Here's how the part is built. I have some questions about the finished solid (model axes, mm). A direction names the side the tool comes from. Coordinates: 2 decimals unless noted, no trailing zeros. Write each loop counter-clockwise with the first axis right and the second up, starting at its lowest first coordinate (ties: lowest second). Pieces come first, ordered by that corner, then holes.
Item 1: If we section it at A-A (x = -8): Please give me the cut outline in (y, z).
Item 2: For faces 5 (the face through (-11, 13, 3.6)), 6 (the face through (9.33, 31.864, 5.215)), 7 (the face through (15, 15, 4)), 8 (the face through (14, -6.48, 0.4)), 9 (the face through (5.75, 13, 2)), which set-ups out of +Z, -Z, +X, -X, +Y, -Y let a thin tool reach every point of the face, with its end or its side?
Item 3: I'm going to push flat-ended pins straight in: pin 1 Ø2 at (y, z) = (33.5, 5) entering from +X; pin 2 Ø1.5 at (x, y) = (9, 25) entering from -Z; pin 3 Ø3 at (y, z) = (33.5, 5) entering from +X. Where does each tip first touch, or does it pass through?
Item 4: If we section it at B-B (y = 7): Please give me the cut outline in (x, z).
Item 5: If I drill on line 1 (X direction, y = 16, z = 1); line 2 (Y direction, x = 8, z = 5); line 3 (X direction, y = 14.5, z = 7), over which ranges is the centre line in solid material (lowest first)?
Item 6: We'd pull the mould along Y, two halves only. Please class faces 1 (the face through (-14.43, -6.9, 3.96)), 2 (the face through (-4, 13, 6)), 3 (the face through (4, 13, 6)), 4 (the face through (-14.5, 14.7, 0.5)): +Y half, -Y half, draft (parallel to the pull), parting line (faces both ways), or undercut.
Item 7: If we section it at C-C (x = 9): Please give me the cut outline in (y, z).
from build123d import *

# Parameters (mm, degrees)
SKETCH1_W           = 30
SKETCH1_H           = 75
BOSS_EXTRUDE1_DEPTH = 8
FILLET2_R           = 2
CUT_EXTRUDE3_DEPTH  = 4.4
CUT_EXTRUDE4_DEPTH  = 4.4
SKETCH11_W          = 30
SKETCH11_H          = 30
CUT_EXTRUDE5_DEPTH  = 29.4
FILLET3_R           = 2
CHAMFER1_SIZE       = 1


with BuildPart() as part:
    # Sketch1 → Boss-Extrude1 (new body)
    with BuildSketch(Plane.XY):
        Rectangle(SKETCH1_W, SKETCH1_H)
    extrude(amount=BOSS_EXTRUDE1_DEPTH)

    # Sketch3 → M4 Tapped Hole1 (revolve, cut)
    with BuildSketch(Plane(origin=(15, 33.5, 5), x_dir=(0, 0, -1), z_dir=(0, 1, 0))):
        Polygon((0, 0), (0, 12.491420021), (1.65, 11.5), (1.65, 0), align=None)
    m4_tapped_hole1 = revolve(axis=Axis((21.35, 33.5, 5), (-1, 0, 0)), mode=Mode.SUBTRACT)

    # Fillet2
    fillet2_edges = [part.edges().sort_by_distance(p)[0] for p in [
        (0, 37.5, 0),
        (0, 37.5, 8),
    ]]
    fillet(fillet2_edges, radius=FILLET2_R)

    # Sketch9 → Cut-Extrude3 (cut)
    with BuildSketch(Plane.XY.offset(8)):
        with BuildLine():
            Line((-12, 0), (-12, 25))
            ThreePointArc((-12, 25), (-8, 29), (-4, 25))
            Line((-4, 25), (-4, 0))
            ThreePointArc((-4, 0), (-8, -4), (-12, 0))
        make_face()
        with BuildLine():
            Line((12, 0), (12, 25))
            ThreePointArc((12, 25), (8, 29), (4, 25))
            Line((4, 25), (4, 0))
            ThreePointArc((4, 0), (8, -4), (12, 0))
        make_face()
    extrude(amount=-CUT_EXTRUDE3_DEPTH, mode=Mode.SUBTRACT)

    # Sketch10 → Cut-Extrude4 (cut)
    with BuildSketch(Plane.XY.offset(3.6)):
        with BuildLine():
            Line((-5.75, 25), (-5.75, 0))
            ThreePointArc((-5.75, 0), (-8, -2.25), (-10.25, 0))
            Line((-10.25, 0), (-10.25, 25))
            ThreePointArc((-10.25, 25), (-8, 27.25), (-5.75, 25))
        make_face()
        with BuildLine():
            Line((5.75, 25), (5.75, 0))
            ThreePointArc((5.75, 0), (8, -2.25), (10.25, 0))
            Line((10.25, 0), (10.25, 25))
            ThreePointArc((10.25, 25), (8, 27.25), (5.75, 25))
        make_face()
    extrude(amount=-CUT_EXTRUDE4_DEPTH, mode=Mode.SUBTRACT)

    # Sketch11 → Cut-Extrude5 (cut)
    with BuildSketch(Plane.XY.offset(8)):
        with Locations((0, -22.5)):
            Rectangle(SKETCH11_W, SKETCH11_H)
    extrude(amount=-CUT_EXTRUDE5_DEPTH, mode=Mode.SUBTRACT)

    # Fillet3
    fillet3_edges = [part.edges().sort_by_distance(p)[0] for p in [
        (15, -7.5, 4),
        (-15, -7.5, 4),
    ]]
    fillet(fillet3_edges, radius=FILLET3_R)

    # Mirror1: M4 Tapped Hole1 across plane
    add(m4_tapped_hole1.mirror(Plane(origin=(0, 0, 0), x_dir=(0, 0, 1), z_dir=(1, 0, 0))), mode=Mode.SUBTRACT)

    # Chamfer1
    chamfer1_edges = [part.edges().sort_by_distance(p)[0] for p in [
        (0, -7.5, 8),
        (0, -7.5, 0),
        (15, 15, 8),
        (-14.414213562, -6.914213562, 8),
        (14.414213562, -6.914213562, 8),
        (15, 15, 0),
        (-14.414213562, -6.914213562, 0),
        (14.414213562, -6.914213562, 0),
        (-15, 37.5, 4),
        (15, 37.5, 4),
        (-15, 15, 0),
        (-15, 15, 8),
        (-15, 36.914213562, 7.414213562),
        (-15, 36.914213562, 0.585786438),
        (15, 36.914213562, 7.414213562),
        (15, 36.914213562, 0.585786438),
    ]]
    chamfer(chamfer1_edges, length=CHAMFER1_SIZE)


solid = part.part
Answer list:
1. outline: (-7.5, 1) - (-6.5, 0) - (-2.25, 0) - (-2.25, 3.6) - (-4, 3.6) - (-4, 8) - (-6.5, 8) - (-7.5, 7) - close; (27.25, 0) - (35.5, 0) arc R2 ccw to (37.5, 2) - (37.5, 6) arc R2 ccw to (35.5, 8) - (29, 8) - (29, 3.6) - (27.25, 3.6) - close; hole circle Ø3.3 at (33.5, 5)
2. face 5: +Z
2. face 6: +X
2. face 7: +Z, -Z, +X, +Y, -Y
2. face 8: -Z, +X, -Y
2. face 9: +Z, -Z
3. pin 1: stops at x = 3.11
3. pin 2: passes through
3. pin 3: stops at x = 3.41
4. outline: (-15, 1) - (-14, 0) - (-10.25, 0) - (-10.25, 3.6) - (-12, 3.6) - (-12, 8) - (-14, 8) - (-15, 7) - close; (-5.75, 0) - (5.75, 0) - (5.75, 3.6) - (4, 3.6) - (4, 8) - (-4, 8) - (-4, 3.6) - (-5.75, 3.6) - close; (10.25, 0) - (14, 0) - (15, 1) - (15, 7) - (14, 8) - (12, 8) - (12, 3.6) - (10.25, 3.6) - close
5. line 1: x = -15 to -10.25, -5.75 to 5.75, 10.25 to 15
5. line 2: y = -7.5 to -4, 29 to 31.85, 35.15 to 37.5
5. line 3: x = -15 to -12, -4 to 4, 12 to 15
6. face 1: -Y half
6. face 2: undercut
6. face 3: undercut
6. face 4: draft
7. outline: (-7.5, 1) - (-6.5, 0) - (-2.02, 0) - (-2.02, 3.6) - (-3.87, 3.6) - (-3.87, 8) - (-6.5, 8) - (-7.5, 7) - close; (27.02, 0) - (35.5, 0) arc R2 ccw to (37.5, 2) - (37.5, 6) arc R2 ccw to (35.5, 8) - (28.87, 8) - (28.87, 3.6) - (27.02, 3.6) - close; hole circle Ø3.3 at (33.5, 5)
